Geometry check sheet. Reference: the model listing, model coordinates, mm. Face numbers are marked on the shaded views. Round coordinates to 2 decimals unless told otherwise and drop trailing zeros. Write each loop counter-clockwise with the first axis right and the second up, starting at its lowest first coordinate (ties: lowest second). Pieces come first, ordered by that corner, then holes.
Item 1: Cross-section at A-A (x = 1). Enter the section's corners in (y, z).
Item 2: Draft check along Y on the marked faces 1, 2 and 3. Enter one of: pulls with the +Y half, pulls with the -Y half, needs draft (parallel to the pull), parting line crosses it, or undercut.
Item 3: Depth check by flat-ended pin: P1, Ø1, axis at x = 1.5, y = -2.5, coming from the +Z side; P2, Ø3, axis at x = 1.5, z = -2.5, coming from the -Y side. Enter the tip coordinate at first touch or a pass-through.
Item 4: Scan lines: probe 1 along Y at (x, z) = (5.25, 0); probe 2 along X at (y, z) = (-2.25, 2.25). Record each from-to range of solid material in increasing order.
Autodesk Inventor part; units mm, degrees
ref_plane "YZ Plane" through (0, 0, 0) normal (1, 0, 0) x (0, 1, 0)
ref_plane "XZ Plane" through (0, 0, 0) normal (0, 1, 0) x (-1, 0, 0)
ref_plane "XY Plane" through (0, 0, 0) normal (0, 0, 1) x (1, 0, 0)
sketch "Skizze1" plane through (0, 0, 0) normal (0, 0, 1) x (1, 0, 0)
  line L0 (7, -3) -> (0, -3)
  line L1 (7, 3) -> (7, -3)
  line L2 (7, 3) -> (0, 3)
  line L3 (7, 1.8) -> (13, 1.8)
  line L4 (7, -1.8) -> (13, -1.8)
  line L5 (0, 3) -> (0, -3)
  line L6 (7, 0) -> (7, 3)
  line L7 (0, 3) -> (-0.1, 3)
  line L8 (-0.1, 3) -> (-0.1, 3.5)
  line L9 (-0.1, 3.5) -> (-0.6, 3.5)
  line L10 (-0.6, 3.5) -> (-0.6, 0)
  line L11 (-0.6, 0) -> (7, 0)
  point P0 (0, 0)
  point P1 (0, 0)
  dimension "d0" = 0.1
  dimension "d1" = 0.5
  dimension "d2" = 0.5
  dimension "d24" = 7.6
  dimension "d25" = 3.5
  dimension "d26" = 3
revolve "Umdrehung1" add sketch "Skizze1" angle 360 about axis through (-0.6, 0, 0) along (1, 0, 0) contours L11 L10 L9 L8 L7 L5 | L5 L2 L1 L11
sketch "Skizze3" plane through (-0.6, 0, 0) normal (-1, 0, 0) x (0, 0, 1)
  point P0 (0, 0)
chamfer "Fase1" distance 0.2 angle 45 1 edges at (7, -3, 0)
chamfer "Fase2" distance 0.2 angle 45 1 edges at (6.8, -3, 0)
hole "Bohrung2" at (-0.6, 0, 0) direction (1, 0, 0) diameter 3 end through all
chamfer "Fase3" distance 0.2 angle 45 1 edges at (-0.6, 0, -1.5)
properties part number "Hülse1"
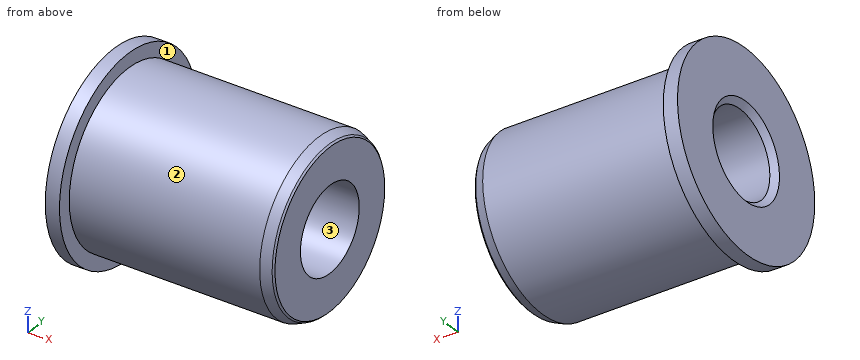
Resolved:
1. outline: circle Ø6 at (0, 0); hole circle Ø3 at (0, 0)
2. face 1: needs draft
2. face 2: parting line crosses it
2. face 3: undercut
3. P1: stops at z = 2.24
3. P2: stops at y = -2.83
4. probe 1: y = -3 to -1.5, 1.5 to 3
4. probe 2: x = -0.6 to -0.1
